```python
from build123d import *

# Parameters (mm, degrees)
SKETCH1_W           = 380
SKETCH1_H           = 285
SKETCH1_R           = 13
SKETCH1_R_2         = 2.125
BOSS_EXTRUDE1_DEPTH = 3.175


with BuildPart() as part:
    # Sketch1 → Boss-Extrude1 (new body)
    with BuildSketch(Plane(origin=(0, 0, 0), x_dir=(1, 0, 0), z_dir=(0, 1, 0))):
        Rectangle(SKETCH1_W, SKETCH1_H)
        with Locations(Location((-95, 39.5, 0), (0, 0, 270))):
            Circle(SKETCH1_R, mode=Mode.SUBTRACT)
        with Locations(Location((-112.5, 39.5, 0), (0, 0, 270))):
            Circle(SKETCH1_R_2, mode=Mode.SUBTRACT)
        with Locations(Location((-47.5, -125, 0), (0, 0, 270))):
            Circle(SKETCH1_R_2, mode=Mode.SUBTRACT)
        with Locations(Location((-47.5, -90, 0), (0, 0, 270))):
            Circle(SKETCH1_R_2, mode=Mode.SUBTRACT)
        with Locations(Location((-95, 57, 0), (0, 0, 270))):
            Circle(SKETCH1_R_2, mode=Mode.SUBTRACT)
        with Locations(Location((-77.5, 39.5, 0), (0, 0, 270))):
            Circle(SKETCH1_R_2, mode=Mode.SUBTRACT)
        with Locations(Location((-95, 22, 0), (0, 0, 270))):
            Circle(SKETCH1_R_2, mode=Mode.SUBTRACT)
        with Locations(Location((-62.5, 132.5, 0), (0, 0, 270))):
            Circle(SKETCH1_R_2, mode=Mode.SUBTRACT)
        with Locations(Location((-62.5, 112.5, 0), (0, 0, 270))):
            Circle(SKETCH1_R_2, mode=Mode.SUBTRACT)
        with Locations(Location((47.5, -90, 0), (0, 0, 90))):
            Circle(SKETCH1_R_2, mode=Mode.SUBTRACT)
        with Locations(Location((47.5, -125, 0), (0, 0, 90))):
            Circle(SKETCH1_R_2, mode=Mode.SUBTRACT)
        with Locations(Location((95, 22, 0), (0, 0, 90))):
            Circle(SKETCH1_R_2, mode=Mode.SUBTRACT)
        with Locations(Location((77.5, 39.5, 0), (0, 0, 90))):
            Circle(SKETCH1_R_2, mode=Mode.SUBTRACT)
        with Locations(Location((112.5, 39.5, 0), (0, 0, 90))):
            Circle(SKETCH1_R_2, mode=Mode.SUBTRACT)
        with Locations(Location((95, 57, 0), (0, 0, 90))):
            Circle(SKETCH1_R_2, mode=Mode.SUBTRACT)
        with Locations(Location((95, 39.5, 0), (0, 0, 90))):
            Circle(SKETCH1_R, mode=Mode.SUBTRACT)
        with Locations(Location((62.5, 112.5, 0), (0, 0, 90))):
            Circle(SKETCH1_R_2, mode=Mode.SUBTRACT)
        with Locations(Location((62.5, 132.5, 0), (0, 0, 90))):
            Circle(SKETCH1_R_2, mode=Mode.SUBTRACT)
        with Locations(Location((-27, -94.5, 0), (0, 0, 270))):
            Circle(SKETCH1_R_2, mode=Mode.SUBTRACT)
        with Locations(Location((-27, -22.5, 0), (0, 0, 270))):
            Circle(SKETCH1_R_2, mode=Mode.SUBTRACT)
        with Locations(Location((27, -94.5, 0), (0, 0, 90))):
            Circle(SKETCH1_R_2, mode=Mode.SUBTRACT)
        with Locations(Location((27, -22.5, 0), (0, 0, 90))):
            Circle(SKETCH1_R_2, mode=Mode.SUBTRACT)
    extrude(amount=BOSS_EXTRUDE1_DEPTH)


solid = part.part
```
The model under review builds one solid part; all positions refer to its coordinate system, in mm. Round coordinates to 2 decimals unless told otherwise and drop trailing zeros.
Item 1: Clearance check with flat-ended pins moving along their axes: pin 1 Ø3.5 at (x, z) = (-62.5, -112.5) entering from +Y; pin 2 Ø7 at (x, z) = (-77.5, -39.5) entering from +Y (3 decimals). State where each tip first meets the part, or that it passes through.
Determined:
pin 1: passes through
pin 2: stops at y = 3.175
Item 2: Mouldability with a two-part tool opening along X and no side actions: class faces 1 (the face through (-3, 3.175, -2)), 2 (the face through (-102.91, 1.565, -49.816)) as released by +X, released by -X, zero draft, split by the parting line, or undercut.
Determined:
face 1: zero draft
face 2: undercut
Item 3: For line 1 (Z direction, x = 95, y = 0.85) (3 decimals); line 2 (X direction, y = 2, z = 90) (3 decimals); line 3 (X direction, y = 1.25, z = -33.5), list the stretches that pass through material, from the lowest coordinate up.
Determined:
line 1: z = -142.5 to -59.125, -54.875 to -52.5, -26.5 to -24.125, -19.875 to 142.5
line 2: x = -190 to -49.625, -45.375 to 45.375, 49.625 to 190
line 3: x = -190 to -106.53, -83.47 to 83.47, 106.53 to 190
